Could you check a few things on this model? Use its own coordinates, in mm. Face numbers are marked on the shaded views. A direction names the side the tool comes from. Round coordinates to 2 decimals unless told otherwise and drop trailing zeros. Loops run counter-clockwise (first coordinate to the right, second up) from the corner with the lowest first, then second, coordinate; pieces in that order, holes last. Notation, with made-up numbers: M -5.75,62.25 L 48.25,62.25 A17 ccw 48.25,91.25 Z; hole C -18,35 d10. An arc over 180 degrees is marked long. Answer in a Markdown table with one row per item.
```python
from build123d import *

# Parameters (mm, degrees)
F0_R     = 5
F1_DEPTH = 13
F2_R     = 16
F2_R_2   = 5
F3_DEPTH = 5
F5_DEPTH = 8
F7_DEPTH = 1


with BuildPart() as f1:
    # F0 (on Top) → F1 (new body)
    with BuildSketch(Plane.XY):
        Circle(F0_R)
        with BuildLine():
            ThreePointArc((1.2, -2.9664793948), (-3.2, 0), (1.2, 2.9664793948))
            Line((1.2, 2.9664793948), (1.2, -2.9664793948))
        make_face(mode=Mode.SUBTRACT)
    extrude(amount=F1_DEPTH)

    # F2 (on face) → F3 (join)
    with BuildSketch(Plane.XY.offset(13)):
        Circle(F2_R)
        Circle(F2_R_2, mode=Mode.SUBTRACT)
        Circle(F2_R_2)
        with BuildLine():
            Line((1.2, 2.9664793948), (1.2, -2.9664793948))
            ThreePointArc((1.2, -2.9664793948), (-3.2, 0), (1.2, 2.9664793948))
        make_face(mode=Mode.SUBTRACT)
        with BuildLine():
            ThreePointArc((1.2, 2.9664793948), (-3.2, 0), (1.2, -2.9664793948))
            Line((1.2, -2.9664793948), (1.2, 2.9664793948))
        make_face()
    extrude(amount=F3_DEPTH)

    # F4 (on face) → F5 (join)
    with BuildSketch(Plane.XY.offset(18)):
        with BuildLine():
            ThreePointArc((4, 15.4919333848), (0, 16), (-4, 15.4919333848))
            Line((-4, 15.4919333848), (-4, -15.4919333848))
            ThreePointArc((-4, -15.4919333848), (0, -16), (4, -15.4919333848))
            Line((4, -15.4919333848), (4, 15.4919333848))
        make_face()
    extrude(amount=F5_DEPTH)

    # F6 (on face) → F7 (join)
    with BuildSketch(Plane.XY.offset(18)):
        with BuildLine():
            Line((-4, 1), (-15.9687194227, 1))
            ThreePointArc((-15.9687194227, 1), (-16, 0), (-15.9687194227, -1))
            Line((-15.9687194227, -1), (-4, -1))
            Line((-4, -1), (-4, 1))
        make_face()
    extrude(amount=F7_DEPTH)


solid = f1.part
```
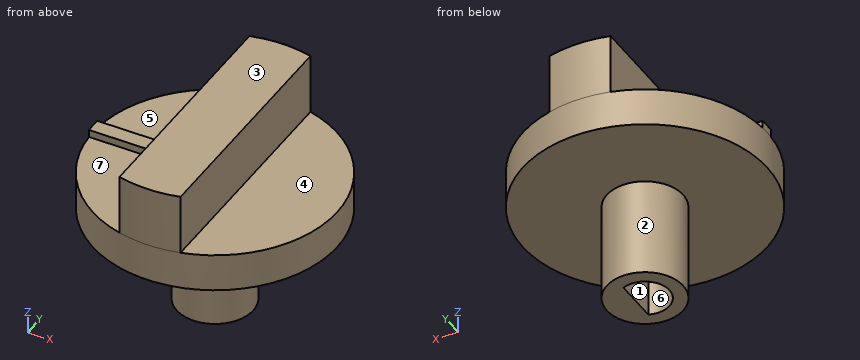
1) Will these pins go through, and if not, where does the flat tip stop? P1, Ø3.5, axis at x = -9.5, y = -6, coming from the +Z side; P2, Ø1.3, axis at x = -0.5, y = 0, coming from the -Z side; P3, Ø2.5, axis at y = 3, z = 22.5, coming from the +X side; P4, Ø5, axis at x = -8, z = 9.5, coming from the -Y side.
Computed:
| item | result |
|---|---|
| P1 | stops at z = 18 |
| P2 | stops at z = 13 |
| P3 | stops at x = 4 |
| P4 | passes through |
2) I want a section at B-B, the plane y = 0. Please give me the cut outline in (x, z), plus the area to 3 significant figures.
Computed:
| item | result |
|---|---|
| outline | M -16,13 L -5,13 L -5,0 L -3.2,0 L -3.2,13 L 1.2,13 L 1.2,0 L 5,0 L 5,13 L 16,13 L 16,18 L 4,18 L 4,26 L -4,26 L -4,19 L -16,19 Z |
| area | 309 mm² |
3) I need wall thicknesses on line 1 (Y direction, x = 0, z = 9); line 2 (Z direction, x = -10, y = -2); line 3 (Z direction, x = 2, y = -9). Which ranges of each line are inside material? Lowest first, please.
Computed:
| item | result |
|---|---|
| line 1 | y = -5 to -3.2, 3.2 to 5 |
| line 2 | z = 13 to 18 |
| line 3 | z = 13 to 26 |
4) I want a section at A-A, the plane x = 0. Please give me the cut outline in (y, z).
Computed:
| item | result |
|---|---|
| outline | M -16,13 L -5,13 L -5,0 L -3.2,0 L -3.2,13 L 3.2,13 L 3.2,0 L 5,0 L 5,13 L 16,13 L 16,26 L -16,26 Z |
5) If we mould it in two halves opening along X, with no side actions, what happens to the marked faces 1, 2 and 3? For each: released by +X, released by -X, zero draft, split by the parting line, or undercut.
Computed:
| item | result |
|---|---|
| face 1 | undercut |
| face 2 | split by the parting line |
| face 3 | zero draft |
6) I want a section at D-D, the plane z = 20.25. Please give me the cut outline in (x, y), plus the area to 3 significant figures.
Computed:
| item | result |
|---|---|
| outline | M -4,-15.49 A16 ccw 4,-15.49 L 4,15.49 A16 ccw -4,15.49 Z |
| area | 253 mm² |
7) Which directions (+Z, -Z, +X, -X, +Y, -Y) give clear straight access to the entire face, cutting with the end or side of a thin tool? Please do the marked faces 4, 5, 6 and 7.
Computed:
| item | result |
|---|---|
| face 4 | +Z, +X, +Y, -Y |
| face 5 | +Z, -X, +Y |
| face 6 | -Z |
| face 7 | +Z, -X, -Y |
8) I want a section at C-C, the plane z = 7.5. Please give me the cut outline in (x, y), plus the area to 3 significant figures.
Computed:
| item | result |
|---|---|
| outline | C 0,0 d10; hole M 1.2,-2.97 L 1.2,2.97 A3.2 ccw long Z |
| area | 55.0 mm² |
